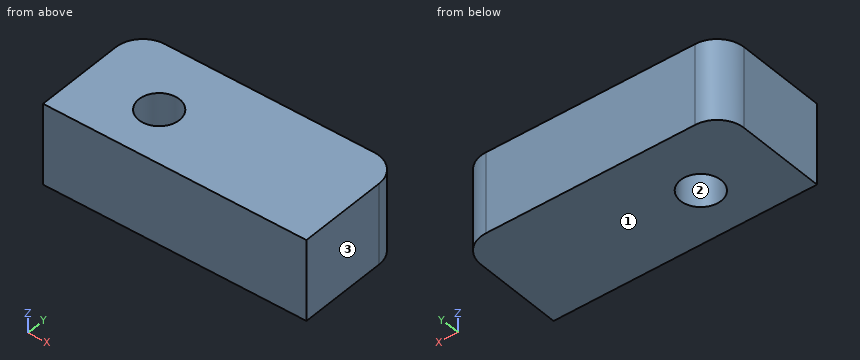
```python
from build123d import *

# Parameters (mm, degrees)
SZKIC1_W                    = 97.5
SZKIC1_H                    = 43
DODANIE_WYCI_GNI_CIE1_DEPTH = 30
ZAOKR_GLENIE1_R             = 10
ZAOKR_GLENIE2_R             = 10
SZKIC2_R                    = 7.5
WYTNIJ_WYCI_GNI_CIE1_DEPTH  = 30


with BuildPart() as part:
    # Szkic1 → Dodanie-wyciągnięcie1 (new body)
    with BuildSketch(Plane.XY):
        Rectangle(SZKIC1_W, SZKIC1_H)
    extrude(amount=DODANIE_WYCI_GNI_CIE1_DEPTH)

    # Zaokrąglenie1
    zaokr_glenie1_edges = [part.edges().sort_by_distance(p)[0] for p in [
        (-48.75, 21.5, 15),
    ]]
    fillet(zaokr_glenie1_edges, radius=ZAOKR_GLENIE1_R)

    # Zaokrąglenie2
    zaokr_glenie2_edges = [part.edges().sort_by_distance(p)[0] for p in [
        (48.75, 21.5, 15),
    ]]
    fillet(zaokr_glenie2_edges, radius=ZAOKR_GLENIE2_R)

    # Szkic2 → Wytnij-wyciągnięcie1 (cut)
    with BuildSketch(Plane.XY.offset(30)):
        with Locations((-21.25, -2.5)):
            Circle(SZKIC2_R)
    extrude(amount=-WYTNIJ_WYCI_GNI_CIE1_DEPTH, mode=Mode.SUBTRACT)


solid = part.part
```
Geometry check sheet. Reference: the model listing, model coordinates, mm. Face numbers are marked on the shaded views. Give positions to 0.01 mm unless a question says otherwise; leave off trailing zeros. Write each loop counter-clockwise with the first axis right and the second up, starting at its lowest first coordinate (ties: lowest second). Pieces come first, ordered by that corner, then holes. Notation, with made-up numbers: (30.25, 48) -> (55.25, 48) arc R18 ccw to (55.25, 67) -> close; hole circle Ø3 at (79.25, 40.25). An arc over 180 degrees is marked (long way). Use one line per item in the form item = value.
Item 1: Depth check by flat-ended pin: pin 1 Ø4 at (x, y) = (23, 0.5) entering from -Z; pin 2 Ø12 at (x, y) = (-21.25, -2.5) entering from +Z. Enter the tip coordinate at first touch or a pass-through.
Results list:
pin_1 = 0
pin_2 = through
Item 2: Sectioned sample at B-B on z = 5. Enter the section's corners in (x, y), plus the area to 3 significant figures.
Results list:
outline = (-48.75, -21.5) -> (48.75, -21.5) -> (48.75, 11.5) arc R10 ccw to (38.75, 21.5) -> (-38.75, 21.5) arc R10 ccw to (-48.75, 11.5) -> close; hole circle Ø15 at (-21.25, -2.5)
area = 3,970 mm2
Item 3: Mould release check, pull along X, two halves, no side actions. Record for the marked faces 1, 2 and 3: released by +X, released by -X, zero draft, split by the parting line, or undercut.
Results list:
face_1 = zero draft
face_2 = undercut
face_3 = released by +X
Item 4: Sectioned sample at D-D on y = 17.5. Enter the section's corners in (x, z), plus the area to 4 significant figures.
Results list:
outline = (-46.75, 0) -> (46.75, 0) -> (46.75, 30) -> (-46.75, 30) -> close
area = 2,805 mm2
Item 5: Scan lines: line 1 (Y direction, x = -21.25, z = 15.25); line 2 (X direction, y = -7, z = 12.75); line 3 (X direction, y = 0, z = 10.5). Record each from-to range of solid material in increasing order.
Results list:
line_1 = -21.5 to -10, 5 to 21.5
line_2 = -48.75 to -27.25, -15.25 to 48.75
line_3 = -48.75 to -28.32, -14.18 to 48.75
Item 6: Sectioned sample at A-A on x = -21.25. Enter the section's corners in (y, z).
Results list:
outline = (-21.5, 0) -> (-10, 0) -> (-10, 30) -> (-21.5, 30) -> close; (5, 0) -> (21.5, 0) -> (21.5, 30) -> (5, 30) -> close
Item 7: Sectioned sample at C-C on y = -2.5. Enter the section's corners in (x, z).
Results list:
outline = (-48.75, 0) -> (-28.75, 0) -> (-28.75, 30) -> (-48.75, 30) -> close; (-13.75, 0) -> (48.75, 0) -> (48.75, 30) -> (-13.75, 30) -> close
